```python
from build123d import *

# Parameters (mm, degrees)
F0_W     = 120
F0_H     = 120
F1_DEPTH = 100
F2_R     = 25
F3_DEPTH = 25


with BuildPart() as f1:
    # F0 (on Top) → F1 (new body)
    with BuildSketch(Plane.XY):
        Rectangle(F0_W, F0_H)
    extrude(amount=F1_DEPTH)


with BuildPart() as f3:
    # F2 (on face) → F3 (new body)
    with BuildSketch(Plane.XY.offset(100)):
        Circle(F2_R)
    extrude(amount=-F3_DEPTH)


with BuildPart() as f1_1:
    add(f1.part)

    # F4: cut F3
    add(f3.part, mode=Mode.SUBTRACT)


solid = f1_1.part
```
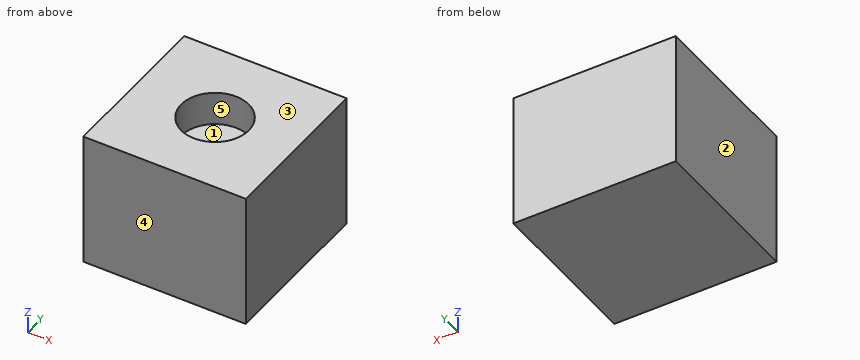
Model file for the job. Use its own axes, mm. Face numbers are marked on the shaded views. A direction names the side the tool comes from. Coordinates: 2 decimals unless noted, no trailing zeros. Order: outer loops, then holes, each group sorted by start corner. A loop starts at its lowest first (then second) coordinate and runs counter-clockwise, first axis right, second up. Notation, with made-up numbers: (33, -20) - (55, -20) arc R16 cw to (55, -1) - close; hole circle Ø8 at (-40, 7). An arc over 180 degrees is marked (long way). Return JSON: item names as keys, results as strings. Group by question number.
1) Saw through at C-C, the plane z = 82.5. Write the cut outline in (x, y).
2) Flat gauge pin, fed straight in: P1, Ø25, axis at x = -4.5, y = -11.5, coming from the +Z side. Where does the tip first touch, or does it go through?
3) Probe line 1 (Y direction, x = 0, z = 88.25); line 2 (Y direction, x = -3.5, z = 77); line 3 (X direction, y = -22, z = 87.5). List the from-to ranges inside material, lowest first. Write a range as from..to.
4) Mould opens along Y. For the marked faces 3, 4 and 5 say: released by +Y, released by -Y, zero draft, split by the parting line, or undercut.
5) Saw through at A-A, the plane x = 0. Write the cut outline in (y, z), plus the area to 4 significant figures.
6) Tool access for the marked faces 1 and 2: list every direction of +Z, -Z, +X, -X, +Y, -Y with a clear straight run to the whole face (end or side of a thin tool).
Values found:
{
 "1": {"outline": "(-60, -60) - (60, -60) - (60, 60) - (-60, 60) - close; hole circle Ø50 at (0, 0)"},
 "2": {"P1": "stops at z = 75"},
 "3": {"line 1": "y = -60..-25, 25..60", "line 2": "y = -60..-24.75, 24.75..60", "line 3": "x = -60..-11.87, 11.87..60"},
 "4": {"face 3": "zero draft", "face 4": "released by -Y", "face 5": "undercut"},
 "5": {"outline": "(-60, 0) - (60, 0) - (60, 100) - (25, 100) - (25, 75) - (-25, 75) - (-25, 100) - (-60, 100) - close", "area": "10,750 mm²"},
 "6": {"face 1": "+Z", "face 2": "+Z, -Z, -X, +Y, -Y"}
}
